Answer from the drawing. Dimensions are ordinates in mm from the lowest x, y and z of the part. Coordinates: 2 decimals unless noted, no trailing zeros. Order: outer loops, then holes, each group sorted by start corner. A loop starts at its lowest first (then second) coordinate and runs counter-clockwise, first axis right, second up. Notation, with made-up numbers: (-19.5, -32) - (38.5, -32) arc R29 cw to (38.5, -9) - close; hole circle Ø11 at (53, 73). An arc over 180 degrees is marked (long way). One line per item, written item: value. Start each with the question number.
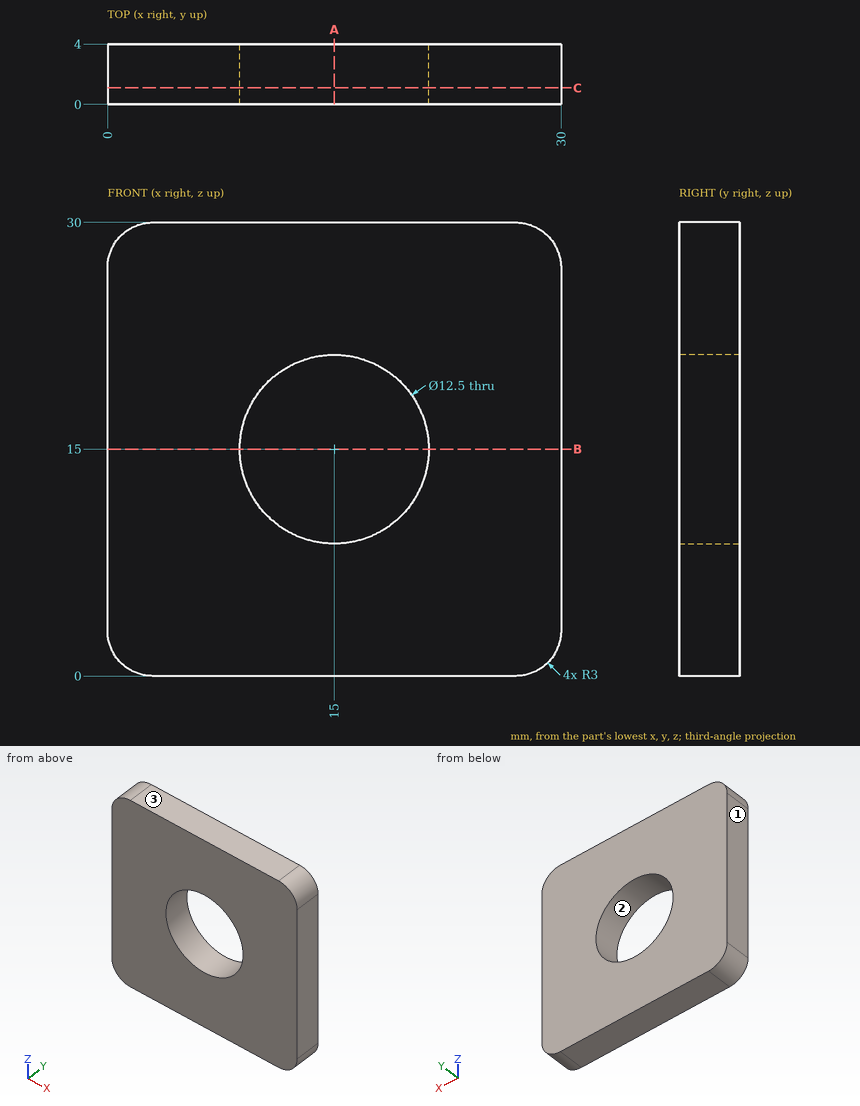
(1) A flat-ended cylindrical pin translates along its axis: pin 1 Ø1 at (x, y) = (18.5, 3.5) entering from -Z. Find the tip coordinate at first contact, or state that the pin passes through.
(2) Consider probe 1 along X at (y, z) = (3.45, 15.25) (3 decimals); probe 2 along Z at (x, y) = (17.25, 3.3); probe 3 along Z at (x, y) = (14, 0.25). Determine where each line is inside the solid, lowest interval first.
(3) For a pull along Z with two mould halves and no side action, classify the marked faces 1, 2 and 3 as pulls with the +Z half, pulls with the -Z half, needs draft (parallel to the pull), parting line crosses it, or undercut.
(4) The part is cut by section A-A on x = 15. Determine the outline of the cut face in (y, z), plus the area to 3 significant figures.
(5) The part is cut by section B-B on z = 15. Determine the outline of the cut face in (x, y), plus the area to 3 significant figures.
(6) The part is cut by section C-C on y = 1.1. Determine the outline of the cut face in (x, z).
Completed:
1. pin 1: stops at z = 0
2. probe 1: x = 0 to 8.755, 21.245 to 30
2. probe 2: z = 0 to 9.17, 20.83 to 30
2. probe 3: z = 0 to 8.83, 21.17 to 30
3. face 1: needs draft
3. face 2: undercut
3. face 3: pulls with the +Z half
4. outline: (0, 0) - (4, 0) - (4, 8.75) - (0, 8.75) - close; (0, 21.25) - (4, 21.25) - (4, 30) - (0, 30) - close
4. area: 70.0 mm2
5. outline: (0, 0) - (8.75, 0) - (8.75, 4) - (0, 4) - close; (21.25, 0) - (30, 0) - (30, 4) - (21.25, 4) - close
5. area: 70.0 mm2
6. outline: (0, 3) arc R3 ccw to (3, 0) - (27, 0) arc R3 ccw to (30, 3) - (30, 27) arc R3 ccw to (27, 30) - (3, 30) arc R3 ccw to (0, 27) - close; hole circle Ø12.5 at (15, 15)
